```python
from build123d import *

# Parameters (mm, degrees)
SKETCH1_W                = 18
SKETCH1_H                = 15
SKETCH1_R                = 2.25
SKETCH1_W_2              = 2.049458383
SKETCH1_H_2              = 2.049458383
SKETCH1_W_3              = 2.049458384
SKETCH1_H_3              = 2.049458384
SKETCH1_W_4              = 2.977571315
SKETCH1_H_4              = 4.783639162
SKETCH1_W_5              = 3.612135694
SKETCH1_H_5              = 3.660948338
SKETCH1_W_6              = 2.855539704
SKETCH1_H_6              = 1.171503468
BOSS_EXTRUDE1_DEPTH      = 1.6
BOSS_EXTRUDE2_DEPTH      = 1.65
BOSS_EXTRUDE2_DEPTH_BACK = 0.05
SKETCH1_3_W              = 2.049458383
SKETCH1_3_H              = 2.049458383
SKETCH1_3_R              = 0.491297767
SKETCH1_3_W_2            = 2.049458384
SKETCH1_3_R_2            = 0.472938465
SKETCH1_3_R_3            = 0.49179988
SKETCH1_3_R_4            = 0.462232329
SKETCH1_3_H_2            = 2.049458384
SKETCH1_3_R_5            = 0.506268972
SKETCH1_4_R              = 2.25
BOSS_EXTRUDE3_DEPTH      = 5
SKETCH1_5_W              = 2.977571315
SKETCH1_5_H              = 4.783639162
SKETCH1_5_W_2            = 2.855539704
SKETCH1_5_H_2            = 1.171503468
SKETCH1_5_W_3            = 3.612135694
SKETCH1_5_H_3            = 3.660948338
BOSS_EXTRUDE4_DEPTH      = 3


with BuildPart() as part:
    # Sketch1 → Boss-Extrude1 (new body)
    with BuildSketch(Plane(origin=(0, 0, 0), x_dir=(1, 0, 0), z_dir=(0, 1, 0))):
        with Locations((438.509935884, 78.243204781)):
            Rectangle(SKETCH1_W, SKETCH1_H)
        with Locations(Location((441.516142154, 83.243204781, 0), (0, 0, 270))):
            Circle(SKETCH1_R, mode=Mode.SUBTRACT)
        with Locations(Location((434.926435145, 83.243204781, 0), (0, 0, 270))):
            Circle(SKETCH1_R, mode=Mode.SUBTRACT)
        with Locations((430.782103127, 83.20757709)):
            Rectangle(SKETCH1_W_2, SKETCH1_H_2, mode=Mode.SUBTRACT)
        with Locations((430.850957935, 80.638087475)):
            Rectangle(SKETCH1_W_3, SKETCH1_H_2, mode=Mode.SUBTRACT)
        with Locations((430.855961247, 73.0772243)):
            Rectangle(SKETCH1_W_2, SKETCH1_H_3, mode=Mode.SUBTRACT)
        with Locations((446.205622618, 83.20757709)):
            Rectangle(SKETCH1_W_2, SKETCH1_H_2, mode=Mode.SUBTRACT)
        with Locations((446.259482022, 73.069490495)):
            Rectangle(SKETCH1_W_2, SKETCH1_H_2, mode=Mode.SUBTRACT)
        with Locations((442.614426656, 77.061445861)):
            Rectangle(SKETCH1_W_4, SKETCH1_H_4, mode=Mode.SUBTRACT)
        with Locations((438.758227739, 73.229653267)):
            Rectangle(SKETCH1_W_5, SKETCH1_H_5, mode=Mode.SUBTRACT)
        with Locations((434.377292894, 72.961183722)):
            Rectangle(SKETCH1_W_6, SKETCH1_H_6, mode=Mode.SUBTRACT)
    extrude(amount=BOSS_EXTRUDE1_DEPTH)

    # Sketch1_3 → Boss-Extrude2 (add, two sides: drawn at the far end of the back side and taken through both)
    # profile 1 of 5: a face of its own
    with BuildSketch(Plane(origin=(0, 0, 0), x_dir=(1, 0, 0), z_dir=(0, 1, 0)).offset(-BOSS_EXTRUDE2_DEPTH_BACK)):
        with Locations((430.782103127, 83.20757709)):
            Rectangle(SKETCH1_3_W, SKETCH1_3_H)
        with Locations(Location((430.842964154, 83.243204781, 0), (0, 0, 270))):
            Circle(SKETCH1_3_R, mode=Mode.SUBTRACT)
    # profile 2 of 5: a face of its own
    with BuildSketch(Plane(origin=(0, 0, 0), x_dir=(1, 0, 0), z_dir=(0, 1, 0)).offset(-BOSS_EXTRUDE2_DEPTH_BACK)):
        with Locations((430.850957935, 80.638087475)):
            Rectangle(SKETCH1_3_W_2, SKETCH1_3_H)
        with Locations(Location((430.842964154, 80.703204781, 0), (0, 0, 270))):
            Circle(SKETCH1_3_R_2, mode=Mode.SUBTRACT)
    # profile 3 of 5: a face of its own
    with BuildSketch(Plane(origin=(0, 0, 0), x_dir=(1, 0, 0), z_dir=(0, 1, 0)).offset(-BOSS_EXTRUDE2_DEPTH_BACK)):
        with Locations((446.205622618, 83.20757709)):
            Rectangle(SKETCH1_3_W, SKETCH1_3_H)
        with Locations(Location((446.243933423, 83.243204781, 0), (0, 0, 270))):
            Circle(SKETCH1_3_R_3, mode=Mode.SUBTRACT)
    # profile 4 of 5: a face of its own
    with BuildSketch(Plane(origin=(0, 0, 0), x_dir=(1, 0, 0), z_dir=(0, 1, 0)).offset(-BOSS_EXTRUDE2_DEPTH_BACK)):
        with Locations((446.259482022, 73.069490495)):
            Rectangle(SKETCH1_3_W, SKETCH1_3_H)
        with Locations(Location((446.243933423, 73.083204781, 0), (0, 0, 270))):
            Circle(SKETCH1_3_R_4, mode=Mode.SUBTRACT)
    # profile 5 of 5: a face of its own
    with BuildSketch(Plane(origin=(0, 0, 0), x_dir=(1, 0, 0), z_dir=(0, 1, 0)).offset(-BOSS_EXTRUDE2_DEPTH_BACK)):
        with Locations((430.855961247, 73.0772243)):
            Rectangle(SKETCH1_3_W, SKETCH1_3_H_2)
        with Locations(Location((430.855961247, 73.083204781, 0), (0, 0, 270))):
            Circle(SKETCH1_3_R_5, mode=Mode.SUBTRACT)
    extrude(amount=BOSS_EXTRUDE2_DEPTH + BOSS_EXTRUDE2_DEPTH_BACK)

    # Sketch1_4 → Boss-Extrude3 (add)
    with BuildSketch(Plane(origin=(0, 0, 0), x_dir=(1, 0, 0), z_dir=(0, 1, 0))):
        with Locations(Location((434.926435145, 83.243204781, 0), (0, 0, 270))):
            Circle(SKETCH1_4_R)
        with Locations(Location((441.516142154, 83.243204781, 0), (0, 0, 270))):
            Circle(SKETCH1_4_R)
    extrude(amount=BOSS_EXTRUDE3_DEPTH)

    # Sketch1_5 → Boss-Extrude4 (add)
    with BuildSketch(Plane(origin=(0, 0, 0), x_dir=(1, 0, 0), z_dir=(0, 1, 0))):
        with Locations((442.614426656, 77.061445861)):
            Rectangle(SKETCH1_5_W, SKETCH1_5_H)
        with Locations((434.377292894, 72.961183722)):
            Rectangle(SKETCH1_5_W_2, SKETCH1_5_H_2)
        with Locations((438.758227739, 73.229653267)):
            Rectangle(SKETCH1_5_W_3, SKETCH1_5_H_3)
    extrude(amount=BOSS_EXTRUDE4_DEPTH)


solid = part.part
```
Check sheet for the modelled part. Datum: model origin and axes. Units: mm. A direction names the side the tool comes from. Round coordinates to 2 decimals unless told otherwise and drop trailing zeros. Order: outer loops, then holes, each group sorted by start corner. A loop starts at its lowest first (then second) coordinate and runs counter-clockwise, first axis right, second up. Notation, with made-up numbers: (14.25, 49) - (28.25, 49) arc R27 ccw to (28.25, 85) - close; hole circle Ø4 at (4, -2.5). An arc over 180 degrees is marked (long way). Write item = value, one per line.
Q1. Section check A-A (y = 2). Record the boundary of the cut face in (x, z).
Computed:
outline = circle Ø4.5 at (434.93, -83.24); (432.95, -73.55) - (435.81, -73.55) - (435.81, -72.38) - (432.95, -72.38) - close; (436.95, -75.06) - (440.56, -75.06) - (440.56, -71.4) - (436.95, -71.4) - close; circle Ø4.5 at (441.52, -83.24); (441.13, -79.45) - (444.1, -79.45) - (444.1, -74.67) - (441.13, -74.67) - close
Q2. Section check B-B (z = -77.5). Record the boundary of the cut face in (x, y), and give its area (3 significant figures).
Computed:
outline = (429.51, 0) - (447.51, 0) - (447.51, 1.6) - (444.1, 1.6) - (444.1, 3) - (441.13, 3) - (441.13, 1.6) - (429.51, 1.6) - close
area = 33.0 mm^2
Q3. Go/stop test with flat-tipped pins: pin 1 (8 mm diameter, centred on x = 444.5, z = -73.5, fed in from +Y); pin 2 (3 mm diameter, centred on x = 441, z = -82.5, fed in from -Y); pin 3 (1 mm diameter, centred on y = 2, z = -80, fed in from +X); pin 4 (1 mm diameter, centred on x = 446.5, z = -73.5, fed in from +Y). Record where each tip stops, or that it passes through.
Computed:
pin_1 = 3
pin_2 = 0
pin_3 = 447.51
pin_4 = 1.65
Q4. Section check C-C (z = -80.5). Record the boundary of the cut face in (x, y).
Computed:
outline = (429.51, 0) - (429.83, 0) - (429.83, -0.05) - (430.42, -0.05) - (430.42, 1.65) - (429.83, 1.65) - (429.83, 1.6) - (429.51, 1.6) - close; (431.27, -0.05) - (431.88, -0.05) - (431.88, 0) - (447.51, 0) - (447.51, 1.6) - (431.88, 1.6) - (431.88, 1.65) - (431.27, 1.65) - close
Q5. Thickness scan on line 1 along X through (y, z) = (0.8, -83.25); line 2 along X through (y, z) = (2.95, -73.5); line 3 along Z through (x, y) = (437.75, 1.95). Record the ranges inside material, lowest first.
Computed:
line_1 = 429.51 to 430.35, 431.33 to 445.75, 446.74 to 447.51
line_2 = 432.95 to 435.81, 436.95 to 440.56
line_3 = -75.06 to -71.4
Q6. Tool access check on faces 1 (the face through (444.103, 2, -77)), 2 (the face through (439, 3, -73)), 3 (the face through (436.952, 2, -73)), 4 (the face through (430, 1.65, -73)), 5 (the face through (443, 2, -79.453)). Record the directions out of +Z, -Z, +X, -X, +Y, -Y that give a thin tool (end or side, any length) a straight path to the whole face; none if there is none.
Computed:
face_1 = +Z, -Z, +X, +Y
face_2 = +Z, +X, -X, +Y
face_3 = +Z, +Y
face_4 = +Z, -Z, -X, +Y
face_5 = +X, -X, +Y
Q7. Section check D-D (x = 442.75). Record the boundary of the cut face in (y, z).
Computed:
outline = (0, -85.74) - (1.6, -85.74) - (1.6, -85.12) - (5, -85.12) - (5, -81.36) - (1.6, -81.36) - (1.6, -79.45) - (3, -79.45) - (3, -74.67) - (1.6, -74.67) - (1.6, -70.74) - (0, -70.74) - close
